Source: CAD feature listing. Evaluate the final solid. Frame: model axes, mm. Face numbers are marked on the shaded views. A direction names the side the tool comes from. Coordinates: 2 decimals unless noted, no trailing zeros. Write each loop counter-clockwise with the first axis right and the second up, starting at its lowest first coordinate (ties: lowest second). Pieces come first, ordered by that corner, then holes. Notation, with made-up numbers: M 80,75.5 L 99,75.5 A14 ccw 99,100.5 Z; hole C -2.75,-32 d10. An arc over 180 degrees is marked long. Answer as CSV lines item,"result". Start each with the question number.
1. Section D-D on x = -5. Return the cut outline in (y, z).
2. Line query: probe 1 along Y at (x, z) = (0, 23.5); probe 2 along Y at (x, z) = (0, 21.15); probe 3 along X at (y, z) = (-8.5, 20.4). Output: solid intervals per line, ascending. Write a range as [from, to].
3. Section B-B on z = 31. Return the cut outline in (x, y), plus the area to 3 significant figures.
4. Section C-C on y = -23. Return the cut outline in (x, z), plus the area to 3 significant figures.
5. Contact query for flat-ended pins moving along their axis: pin 1 Ø10 at (y, z) = (-15.5, 12.5) entering from +X; pin 2 Ø2.5 at (x, z) = (3, 21) entering from +Y; pin 3 Ø1 at (x, z) = (-25, 5.5) entering from +Y. Output: stop coordinate, or through.
6. Mould query, pull axis X, two halves, no side actions, for the marked faces 3, 4 and 5. Classes: pulls with the +X half, pulls with the -X half, needs draft (parallel to the pull), parting line crosses it, or undercut.
7. Section A-A on x = 25. Return the cut outline in (y, z), plus the area to 3 significant figures.
8. Reachability of the marked faces 1 and 2 from +Z, -Z, +X, -X, +Y, -Y: full face, straight path, thin tool, end or side. Return the list, or none.
```python
from build123d import *

# Parameters (mm, degrees)
SKETCH1_R                       = 40.25
BOSS_EXTRUDE1_DEPTH             = 23
SKETCH2_R                       = 12
CUT_EXTRUDE1_DEPTH              = 1
BOSS_EXTRUDE2_START             = 1
SKETCH3_R                       = 13
SKETCH3_R_2                     = 12
BOSS_EXTRUDE2_DEPTH             = 1
SKETCH4_R                       = 6.75
BOSS_EXTRUDE3_DEPTH             = 2
SKETCH7_R                       = 4
BOSS_EXTRUDE5_DEPTH             = 1
BOSS_EXTRUDE6_DEPTH             = 11
SKETCH8_R                       = 4
BOSS_EXTRUDE7_DEPTH             = 4
CUT_EXTRUDE2_START              = -0.2
SKETCH9_R                       = 40.25
SKETCH9_R_2                     = 39.25
CUT_EXTRUDE2_DEPTH              = 0.2
CUT_EXTRUDE4_START              = -0.2
CUT_EXTRUDE4_DEPTH              = 0.2
CUT_EXTRUDE5_START              = -3
CUT_EXTRUDE5_DEPTH              = 3
F_4_0MM_DOWEL_HOLE1_D           = 4
F_4_0MM_DOWEL_HOLE1_DEPTH       = 5.5
F_4_0MM_DOWEL_HOLE1_CSINK_D     = 4.05
F_4_0MM_DOWEL_HOLE1_CSINK_ANGLE = 90
F_4_0MM_DOWEL_HOLE1_TIP         = 1.201721238


with BuildPart() as part:
    # Sketch1 → Boss-Extrude1 (new body)
    with BuildSketch(Plane.XY):
        Circle(SKETCH1_R)
    extrude(amount=BOSS_EXTRUDE1_DEPTH)

    # Sketch2 → Cut-Extrude1 (cut)
    with BuildSketch(Plane.XY.offset(23)):
        Circle(SKETCH2_R)
    extrude(amount=-CUT_EXTRUDE1_DEPTH, mode=Mode.SUBTRACT)

    # Sketch3 → Boss-Extrude2 (add)
    with BuildSketch(Plane.XY.offset(23).offset(BOSS_EXTRUDE2_START)):
        Circle(SKETCH3_R)
        Circle(SKETCH3_R_2, mode=Mode.SUBTRACT)
    extrude(amount=-BOSS_EXTRUDE2_DEPTH)

    # Sketch4 → Boss-Extrude3 (add)
    with BuildSketch(Plane.XY.offset(22)):
        Circle(SKETCH4_R)
    extrude(amount=BOSS_EXTRUDE3_DEPTH)

    # Sketch7 → Boss-Extrude5 (add)
    with BuildSketch(Plane.XY.offset(24)):
        Circle(SKETCH7_R)
    extrude(amount=BOSS_EXTRUDE5_DEPTH)

    # Sketch5 → Boss-Extrude6 (add)
    with BuildSketch(Plane.XY.offset(24)):
        with BuildLine():
            Line((0, 0), (0, -4))
            ThreePointArc((0, -4), (2.828427125, -2.828427125), (4, 0))
            Line((4, 0), (0, 0))
        make_face()
        with BuildLine():
            Line((0, 3.4), (0, 0))
            Line((0, 0), (4, 0))
            ThreePointArc((4, 0), (3.494890771, 1.945697433), (2.107130751, 3.4))
            Line((2.107130751, 3.4), (0, 3.4))
        make_face()
        with BuildLine():
            Line((-3.4, 0), (0, 0))
            Line((0, 0), (0, 3.4))
            Line((0, 3.4), (-2.107130751, 3.4))
            ThreePointArc((-2.107130751, 3.4), (-2.828427125, 2.828427125), (-3.4, 2.107130751))
            Line((-3.4, 2.107130751), (-3.4, 0))
        make_face()
        with BuildLine():
            ThreePointArc((-3.4, -2.107130751), (-1.945697433, -3.494890771), (0, -4))
            Line((0, -4), (0, 0))
            Line((0, 0), (-3.4, 0))
            Line((-3.4, 0), (-3.4, -2.107130751))
        make_face()
    extrude(amount=BOSS_EXTRUDE6_DEPTH)

    # Sketch8 → Boss-Extrude7 (add)
    with BuildSketch(Plane.XY.offset(35)):
        Circle(SKETCH8_R)
    extrude(amount=BOSS_EXTRUDE7_DEPTH)

    # Sketch9 → Cut-Extrude2 (cut)
    with BuildSketch(Plane.XY.offset(23).offset(CUT_EXTRUDE2_START)):
        Circle(SKETCH9_R)
        Circle(SKETCH9_R_2, mode=Mode.SUBTRACT)
    extrude(amount=CUT_EXTRUDE2_DEPTH, mode=Mode.SUBTRACT)

    # Sketch11 → Cut-Extrude4 (cut)
    with BuildSketch(Plane.XY.offset(23).offset(CUT_EXTRUDE4_START)):
        with BuildLine():
            ThreePointArc((6.75, 38.665229858), (3.387641367, 39.103534188), (0, 39.25))
            Line((0, 39.25), (0, 35.25))
            Line((0, 35.25), (6.75, 35.25))
            Line((6.75, 35.25), (6.75, 38.665229858))
        make_face()
        with BuildLine():
            Line((0, 35.25), (0, 39.25))
            ThreePointArc((0, 39.25), (-3.387641367, 39.103534188), (-6.75, 38.665229858))
            Line((-6.75, 38.665229858), (-6.75, 35.25))
            Line((-6.75, 35.25), (0, 35.25))
        make_face()
    extrude(amount=CUT_EXTRUDE4_DEPTH, mode=Mode.SUBTRACT)

    # Sketch12 → Cut-Extrude5 (cut)
    with BuildSketch(Plane.XY.offset(22.8).offset(CUT_EXTRUDE5_START)):
        with BuildLine():
            Line((-6.75, 38.25), (6.75, 38.25))
            Line((6.75, 38.25), (6.75, 38.665229858))
            Line((6.75, 38.665229858), (6.75, 39.679969758))
            ThreePointArc((6.75, 39.679969758), (3.820610596, 40.068259691), (0.870628209, 40.24058283))
            Line((0.870628209, 40.24058283), (-0.870628209, 40.24058283))
            ThreePointArc((-0.870628209, 40.24058283), (-3.820610596, 40.068259691), (-6.75, 39.679969758))
            Line((-6.75, 39.679969758), (-6.75, 38.665229858))
            Line((-6.75, 38.665229858), (-6.75, 38.25))
        make_face()
        with BuildLine():
            Line((-0.870628209, 40.24058283), (0.870628209, 40.24058283))
            ThreePointArc((0.870628209, 40.24058283), (0, 40.25), (-0.870628209, 40.24058283))
        make_face()
    extrude(amount=CUT_EXTRUDE5_DEPTH, mode=Mode.SUBTRACT)

    # Ø4.0mm Dowel Hole1
    with Locations(Plane.XY.offset(23)):
        with Locations((0, 17), (14.722431864, -8.5), (-14.722431864, -8.5)):
            CounterSinkHole(F_4_0MM_DOWEL_HOLE1_D / 2, F_4_0MM_DOWEL_HOLE1_CSINK_D / 2, depth=F_4_0MM_DOWEL_HOLE1_DEPTH, counter_sink_angle=F_4_0MM_DOWEL_HOLE1_CSINK_ANGLE)
            with Locations((0, 0, -(F_4_0MM_DOWEL_HOLE1_DEPTH + F_4_0MM_DOWEL_HOLE1_TIP / 2))):  # 118° drill point
                Cone(0, F_4_0MM_DOWEL_HOLE1_D / 2, F_4_0MM_DOWEL_HOLE1_TIP, mode=Mode.SUBTRACT)


solid = part.part
```
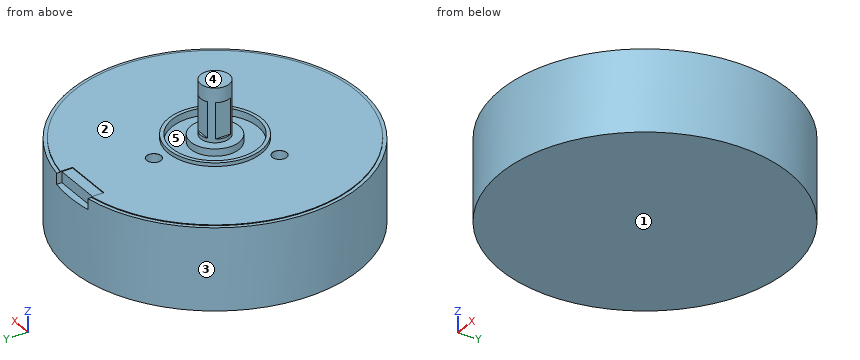
Values:
1,outline,"M -39.94,0 L 39.94,0 L 39.94,19.8 L 38.25,19.8 L 38.25,22.8 L 35.25,22.8 L 35.25,23 L 12,23 L 12,24 L 10.91,24 L 10.91,22 L 4.53,22 L 4.53,24 L -4.53,24 L -4.53,22 L -10.91,22 L -10.91,24 L -12,24 L -12,23 L -38.93,23 L -38.93,22.8 L -39.94,22.8 Z"
2,probe 1,"[-13, -12], [-6.75, 6.75], [12, 13]"
2,probe 2,"[-40.25, 15], [19, 38.25]"
2,probe 3,"[-39.34, -16.72], [-12.72, 12.72], [16.72, 39.34]"
3,outline,"M -3.4,-2.11 A4 ccw long 2.11,3.4 L -2.11,3.4 A4 ccw -3.4,2.11 Z"
3,area,"46.8 mm²"
4,outline,"M -33.03,0 L 33.03,0 L 33.03,22.8 L 31.81,22.8 L 31.81,23 L -31.81,23 L -31.81,22.8 L -33.03,22.8 Z"
4,area,"1,520 mm²"
5,pin 1,"x = 38.86"
5,pin 2,"y = 40.16"
5,pin 3,"y = 31.93"
6,face 3,"parting line crosses it"
6,face 4,"needs draft"
6,face 5,"undercut"
7,outline,"M -31.54,0 L 31.54,0 L 31.54,22.8 L 30.26,22.8 L 30.26,23 L -30.26,23 L -30.26,22.8 L -31.54,22.8 Z"
7,area,"1,450 mm²"
8,face 1,"-Z, +X, -X, +Y, -Y"
8,face 2,"+Z"
